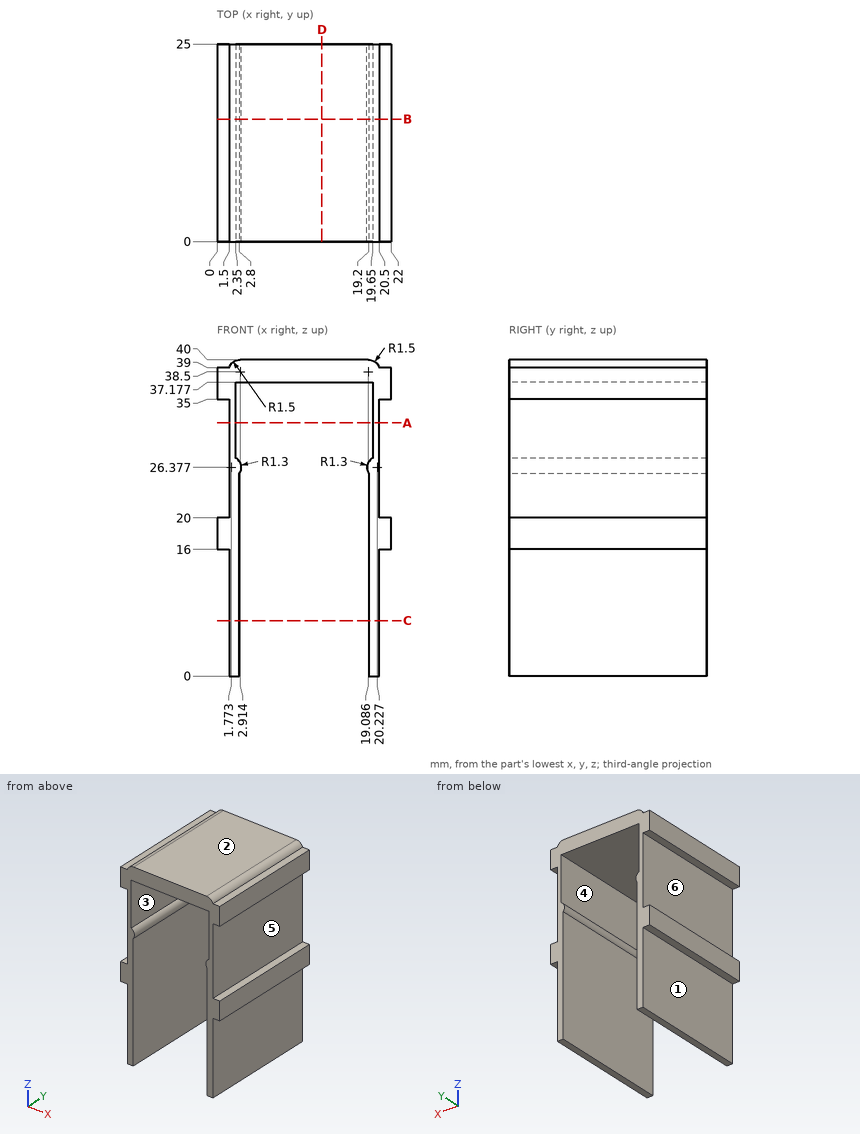
Can you work these out from the drawing? Everything is in mm from the part's minimum corner. A direction names the side the tool comes from. Coordinates: 2 decimals unless noted, no trailing zeros. Loops run counter-clockwise (first coordinate to the right, second up) from the corner with the lowest first, then second, coordinate; pieces in that order, holes last.
1. For the marked faces 4, 5 and 6, which set-ups out of +Z, -Z, +X, -X, +Y, -Y let a thin tool reach every point of the face, with its end or its side?
2. For P1, Ø12.5, axis at y = 15, z = 9, coming from the +X side; P2, Ø2, axis at y = 12, z = 9, coming from the -X side; P3, Ø0.8, axis at x = 21.5, y = 15, coming from the +Z side; P4, Ø6, axis at x = 8.5, z = 28, coming from the -Y side, each with a flat end and sliding along its axis, tell me the tip position at first contact or that it passes through.
3. I need wall thicknesses on L1, parallel to X at y = 18.5, z = 28; L2, parallel to X at y = 1.5, z = 11.5; L3, parallel to Z at x = 10, y = 24. Which ranges of each line are inside material? Lowest first, please.
4. Imagine slicing it at D-D, the plane x = 13.25. Please give me the cut outline in (y, z).
5. Imagine slicing it at A-A, the plane z = 32. Please give me the cut outline in (x, y).
6. Imagine slicing it at B-B, the plane y = 15.5. Please give me the cut outline in (x, z).
7. If we mould it in two halves opening along Z, with no side actions, what happens to the marked faces 1, 2 and 3? For each: pulls with the +Z half, pulls with the -Z half, needs draft (parallel to the pull), parting line crosses it, or undercut.
8. Imagine slicing it at C-C, the plane z = 7. Please give me the cut outline in (x, y).
Taken from the geometry:
1. face 4: +Y, -Y
1. face 5: +X, +Y, -Y
1. face 6: -X, +Y, -Y
2. P1: stops at x = 20.5
2. P2: stops at x = 1.5
2. P3: stops at z = 39
2. P4: passes through
3. L1: x = 1.5 to 2.35, 19.65 to 20.5
3. L2: x = 1.5 to 2.8, 19.2 to 20.5
3. L3: z = 37.18 to 40
4. outline: (0, 37.18) - (25, 37.18) - (25, 40) - (0, 40) - close
5. outline: (1.5, 0) - (2.35, 0) - (2.35, 25) - (1.5, 25) - close; (19.65, 0) - (20.5, 0) - (20.5, 25) - (19.65, 25) - close
6. outline: (0, 16) - (1.5, 16) - (1.5, 0) - (2.8, 0) - (2.8, 25.58) arc R1.3 ccw to (2.35, 27.54) - (2.35, 37.18) - (19.65, 37.18) - (19.65, 27.54) arc R1.3 ccw to (19.2, 25.58) - (19.2, 0) - (20.5, 0) - (20.5, 16) - (22, 16) - (22, 20) - (20.5, 20) - (20.5, 35) - (22, 35) - (22, 39) - (20.5, 39) arc R1.5 ccw to (19.09, 40) - (2.91, 40) arc R1.5 ccw to (1.5, 39) - (0, 39) - (0, 35) - (1.5, 35) - (1.5, 20) - (0, 20) - close
7. face 1: needs draft
7. face 2: pulls with the +Z half
7. face 3: undercut
8. outline: (1.5, 0) - (2.8, 0) - (2.8, 25) - (1.5, 25) - close; (19.2, 0) - (20.5, 0) - (20.5, 25) - (19.2, 25) - close
